from build123d import *

# Parameters (mm, degrees)
F1_ANGLE  = 180
F2_R      = 11
F3_DEPTH  = 3.5
F4_R      = 10.5
F5_DEPTH  = 17
F7_DEPTH  = 4
F8_R      = 18.641205443
F8_R_2    = 11
F9_DEPTH  = 4
F10_R     = 10
F11_DEPTH = 2
F13_DEPTH = 3
F15_DEPTH = 25
F17_DEPTH = 3
F18_R     = 2.5
F19_DEPTH = 2.5
F20_R     = 1.5
F21_DEPTH = 25


with BuildPart() as f1:
    # F0 (on Top) → F1 (revolve)
    with BuildSketch(Plane.XY):
        with BuildLine():
            ThreePointArc((0, -17.5), (12.3743686708, -12.3743686708), (17.5, 0))
            ThreePointArc((17.5, 0), (12.3743686708, 12.3743686708), (0, 17.5))
            Line((0, 17.5), (0, -17.5))
        make_face()
    revolve(axis=Axis((0, 0, 0), (0, -1, 0)), revolution_arc=F1_ANGLE)

    # F2 (on face) → F3 (cut)
    with BuildSketch(Plane(origin=(0, 0, 0), x_dir=(1, 0, 0), z_dir=(0, 0, -1))):
        Circle(F2_R)
    extrude(amount=-F3_DEPTH, mode=Mode.SUBTRACT)

    # F4 (on face) → F5 (cut)
    with BuildSketch(Plane(origin=(0, 0, 3.5), x_dir=(1, 0, 0), z_dir=(0, 0, -1))):
        Circle(F4_R)
    extrude(amount=-F5_DEPTH, mode=Mode.SUBTRACT)



with BuildPart() as f7:
    # F6 (on face) → F7 (new body)
    with BuildSketch(Plane(origin=(0, 0, 0), x_dir=(1, 0, 0), z_dir=(0, 0, -1))):
        with BuildLine():
            ThreePointArc((-12.3743686708, -12.3743686708), (-17.5, 0), (-12.3743686708, 12.3743686708))
            Line((-12.3743686708, 12.3743686708), (-14.1421356237, 14.1421356237))
            ThreePointArc((-14.1421356237, 14.1421356237), (-27.8923182516, 7.317919876), (-43.1821195756, 8.6815247843))
            Line((-43.1821195756, 8.6815247843), (-48.919726111, 4.6715533074))
            ThreePointArc((-48.919726111, 4.6715533074), (-34.6649635656, -10.5286316429), (-14.1421356237, -14.1421356237))
            Line((-14.1421356237, -14.1421356237), (-12.3743686708, -12.3743686708))
        make_face()
        with BuildLine():
            Line((-14.1421356237, 14.1421356237), (-12.3743686708, 12.3743686708))
            ThreePointArc((-12.3743686708, 12.3743686708), (0, 17.5), (12.3743686708, 12.3743686708))
            Line((12.3743686708, 12.3743686708), (14.1421356237, 14.1421356237))
            ThreePointArc((14.1421356237, 14.1421356237), (7.317919876, 27.8923182516), (8.6815247843, 43.1821195756))
            Line((8.6815247843, 43.1821195756), (4.6715533074, 48.919726111))
            ThreePointArc((4.6715533074, 48.919726111), (-10.5286316429, 34.6649635656), (-14.1421356237, 14.1421356237))
        make_face()
        with BuildLine():
            Line((14.1421356237, 14.1421356237), (12.3743686708, 12.3743686708))
            ThreePointArc((12.3743686708, 12.3743686708), (17.5, 0), (12.3743686708, -12.3743686708))
            Line((12.3743686708, -12.3743686708), (14.1421356237, -14.1421356237))
            ThreePointArc((14.1421356237, -14.1421356237), (27.8923182516, -7.317919876), (43.1821195756, -8.6815247843))
            Line((43.1821195756, -8.6815247843), (48.919726111, -4.6715533074))
            ThreePointArc((48.919726111, -4.6715533074), (34.6649635656, 10.5286316429), (14.1421356237, 14.1421356237))
        make_face()
        with BuildLine():
            ThreePointArc((12.3743686708, -12.3743686708), (0, -17.5), (-12.3743686708, -12.3743686708))
            Line((-12.3743686708, -12.3743686708), (-14.1421356237, -14.1421356237))
            ThreePointArc((-14.1421356237, -14.1421356237), (-7.317919876, -27.8923182516), (-8.6815247843, -43.1821195756))
            Line((-8.6815247843, -43.1821195756), (-4.6715533074, -48.919726111))
            ThreePointArc((-4.6715533074, -48.919726111), (10.5286316429, -34.6649635656), (14.1421356237, -14.1421356237))
            Line((14.1421356237, -14.1421356237), (12.3743686708, -12.3743686708))
        make_face()
    extrude(amount=-F7_DEPTH)


with BuildPart() as f1_1:
    add(f1.part)

    add(f7.part)  # F9 merges F7
    # F8 (on face) → F9 (join, through all)
    with BuildSketch(Plane(origin=(0, 0, 0), x_dir=(1, 0, 0), z_dir=(0, 0, -1))):
        Circle(F8_R)
        Circle(F8_R_2, mode=Mode.SUBTRACT)
    extrude(amount=-F9_DEPTH)

    # F10 (on face) → F11 (cut)
    with BuildSketch(Plane(origin=(0, 0, 0), x_dir=(1, 0, 0), z_dir=(0, 0, -1))):
        with Locations((-3.7499996834, 22.8846166283)):
            Circle(F10_R)
        with Locations((-22.8846166283, -3.7499996834)):
            Circle(F10_R)
        with Locations((3.7499996834, -22.8846166283)):
            Circle(F10_R)
        with Locations((22.8846166283, 3.7499996834)):
            Circle(F10_R)
    extrude(amount=-F11_DEPTH, mode=Mode.SUBTRACT)

    # F12 (on face) → F13 (cut)
    with BuildSketch(Plane(origin=(0, 0, 0), x_dir=(1, 0, 0), z_dir=(0, 0, -1))):
        Polygon((5.9440483259, 41.5129213729), (8.2390909401, 43.1169099636), (4.9165431449, 47.8709268072), (2.6215005308, 46.2669382165), (2.2936373002, 46.0377969892), (5.6161850953, 41.2837801456), align=None)
        Polygon((-46.0377969892, 2.2936373002), (-41.2837801456, 5.6161850953), (-41.5129213729, 5.9440483259), (-43.1169099636, 8.2390909401), (-47.8709268072, 4.9165431449), (-46.2669382165, 2.6215005308), align=None)
        Polygon((-2.2936373002, -46.0377969892), (-5.6161850953, -41.2837801456), (-5.9440483259, -41.5129213729), (-8.2390909401, -43.1169099636), (-4.9165431449, -47.8709268072), (-2.6215005308, -46.2669382165), align=None)
        Polygon((46.0377969892, -2.2936373002), (41.2837801456, -5.6161850953), (41.5129213729, -5.9440483259), (43.1169099636, -8.2390909401), (47.8709268072, -4.9165431449), (46.2669382165, -2.6215005308), align=None)
    extrude(amount=-F13_DEPTH, mode=Mode.SUBTRACT)

    # F14 (on face) → F15 (cut)
    with BuildSketch(Plane(origin=(0, 0, 0), x_dir=(1, 0, 0), z_dir=(0, 0, -1))):
        Polygon((5.7307557089, 41.1198485303), (2.2936373002, 46.0377969892), (2.20770934, 46.1607457007), (0.9782222253, 45.3014660985), (4.415340634, 40.3835176396), (4.5012685942, 40.2605689282), align=None)
        Polygon((-46.1607457007, 2.20770934), (-45.3014660985, 0.9782222253), (-40.3835176396, 4.415340634), (-40.2605689282, 4.5012685942), (-41.1198485303, 5.7307557089), (-46.0377969892, 2.2936373002), align=None)
        Polygon((-2.20770934, -46.1607457007), (-0.9782222253, -45.3014660985), (-4.415340634, -40.3835176396), (-4.5012685942, -40.2605689282), (-5.7307557089, -41.1198485303), (-2.2936373002, -46.0377969892), align=None)
        Polygon((46.1607457007, -2.20770934), (45.3014660985, -0.9782222253), (40.3835176396, -4.415340634), (40.2605689282, -4.5012685942), (41.1198485303, -5.7307557089), (46.0377969892, -2.2936373002), align=None)
    extrude(amount=-F15_DEPTH, mode=Mode.SUBTRACT)

    # F16 (on face) → F17 (cut)
    with BuildSketch(Plane(origin=(0, 0, 0), x_dir=(1, 0, 0), z_dir=(0, 0, -1))):
        with BuildLine():
            Line((4.1809628018, 40.7188735865), (1.342054472, 44.7808822767))
            ThreePointArc((1.342054472, 44.7808822767), (-5.3985401919, 39.5803016206), (-8.5350042844, 31.6654896468))
            ThreePointArc((-8.5350042844, 31.6654896468), (-4.3224338027, 32.8682191434), (0, 32.1548648652))
            ThreePointArc((0, 32.1548648652), (1.0537931887, 36.9429820748), (4.1809628018, 40.7188735865))
        make_face()
        with BuildLine():
            Line((-40.7188735865, 4.1809628018), (-44.7808822767, 1.342054472))
            ThreePointArc((-44.7808822767, 1.342054472), (-39.5803016206, -5.3985401919), (-31.6654896468, -8.5350042844))
            ThreePointArc((-31.6654896468, -8.5350042844), (-32.8682191434, -4.3224338027), (-32.1548648653, 0))
            ThreePointArc((-32.1548648653, 0), (-36.9429820748, 1.0537931887), (-40.7188735865, 4.1809628018))
        make_face()
        with BuildLine():
            Line((-4.1809628018, -40.7188735865), (-1.342054472, -44.7808822767))
            ThreePointArc((-1.342054472, -44.7808822767), (5.3985401919, -39.5803016206), (8.5350042844, -31.6654896468))
            ThreePointArc((8.5350042844, -31.6654896468), (4.3224338027, -32.8682191434), (0, -32.1548648653))
            ThreePointArc((0, -32.1548648653), (-1.0537931887, -36.9429820748), (-4.1809628018, -40.7188735865))
        make_face()
        with BuildLine():
            Line((40.7188735865, -4.1809628018), (44.7808822767, -1.342054472))
            ThreePointArc((44.7808822767, -1.342054472), (39.5803016206, 5.3985401919), (31.6654896468, 8.5350042844))
            ThreePointArc((31.6654896468, 8.5350042844), (32.8682191434, 4.3224338027), (32.1548648652, 0))
            ThreePointArc((32.1548648652, 0), (36.9429820748, -1.0537931887), (40.7188735865, -4.1809628018))
        make_face()
    extrude(amount=-F17_DEPTH, mode=Mode.SUBTRACT)

    # F18 (on face) → F19 (join)
    with BuildSketch(Plane(origin=(0, 0, 0), x_dir=(1, 0, 0), z_dir=(0, 0, -1))):
        with Locations((8.4528671578, 13.4043414146)):
            Circle(F18_R)
        with Locations((-13.4043414146, 8.4528671578)):
            Circle(F18_R)
        with Locations((-8.4528671578, -13.4043414146)):
            Circle(F18_R)
        with Locations((13.4043414146, -8.4528671578)):
            Circle(F18_R)
    extrude(amount=F19_DEPTH)

    # F20 (on face) → F21 (cut)
    with BuildSketch(Plane(origin=(0, 0, 0), x_dir=(1, 0, 0), z_dir=(0, 0, -1))):
        with Locations((4.0849614888, 34.4008803368)):
            Circle(F20_R)
        with Locations((-34.4008803368, 4.0849614888)):
            Circle(F20_R)
        with Locations((-4.0849614888, -34.4008803368)):
            Circle(F20_R)
        with Locations((34.4008803368, -4.0849614888)):
            Circle(F20_R)
    extrude(amount=-F21_DEPTH, mode=Mode.SUBTRACT)


solid = f1_1.part
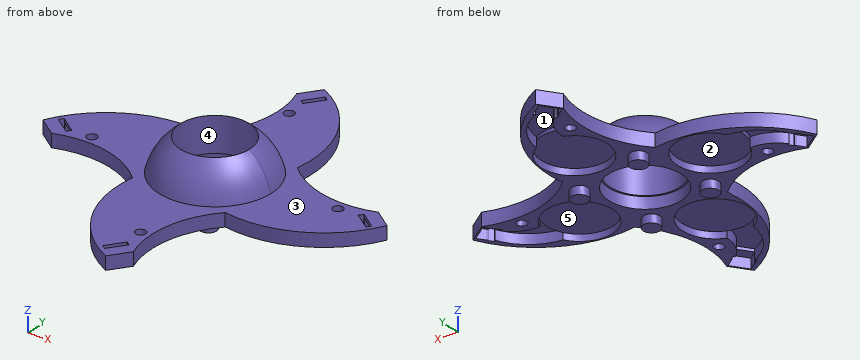
Here's how the part is built. I have some questions about the finished solid (model axes, mm). Face numbers are marked on the shaded views. A direction names the side the tool comes from. Coordinates: 2 decimals unless noted, no trailing zeros. Write each loop counter-clockwise with the first axis right and the second up, starting at its lowest first coordinate (ties: lowest second). Pieces come first, ordered by that corner, then holes.
1) Thinking about a two-plate mould opening in Y: for the marked faces 1, 2 and 3, which applies, +Y half, -Y half, draft (parallel to the pull), parting line (faces both ways), or undercut?
Filled in:
face 1: undercut
face 2: undercut
face 3: draft
2) I'm going to push flat-ended pins straight in: pin 1 (14 mm diameter, centred on x = -36, y = 4, fed in from -Z); pin 2 (8 mm diameter, centred on x = -33.5, z = 9, fed in from +Y); pin 3 (1.5 mm diameter, centred on x = -12.5, y = 11, fed in from +Z); pin 4 (5 mm diameter, centred on x = 4.08, y = -34.4, fed in from +Z). Where does each tip first touch, or does it pass through?
Filled in:
pin 1: stops at z = 0
pin 2: passes through
pin 3: stops at z = 7.31
pin 4: stops at z = 4
3) If we section it at B-B (y = 22): List the corners of the cut face in (x, z) for me.
Filled in:
outline: (-9.11, 0) - (-6.21, 0) - (-6.21, 2) - (13.71, 2) - (13.71, 0) - (14.36, 0) - (14.36, 4) - (-9.11, 4) - close
4) If I drill on line 1 (Y direction, x = 2.5, z = 1.75); line 2 (Z direction, x = 9.5, y = -21); line 3 (X direction, y = 3.75, z = 1.45), over which ranges is the centre line in solid material (lowest first)?
Filled in:
line 1: y = -47.82 to -46.18, -39.15 to -30.69, -15.08 to -10.71, 10.71 to 12.96, 42.54 to 44.42
line 2: z = 0 to 4
line 3: x = -43.33 to -41.45, -12.88 to -10.34, 10.34 to 16.27, 29.5 to 32.94, 35.86 to 40.38, 47.06 to 48.48
5) If we section it at D-D (z = 5.5): List the corners of the cut face in (x, y) for me, plus the area to 3 significant figures.
Filled in:
outline: circle Ø33.23 at (0, 0); hole circle Ø21 at (0, 0)
area: 521 mm2
6) If we section it at C-C (z = 11.5): List the corners of the cut face in (x, y) for me.
Filled in:
outline: circle Ø26.38 at (0, 0); hole circle Ø21 at (0, 0)
7) Which directions (+Z, -Z, +X, -X, +Y, -Y) give clear straight access to the entire face, cutting with the end or side of a thin tool? Please do the marked faces 4 and 5.
Filled in:
face 4: +Z, -Z
face 5: -Z
8) If we section it at A-A (x = -29.5): List the corners of the cut face in (y, z) for me, plus the area to 3 significant figures.
Filled in:
outline: (-7.06, 0) - (-3.75, 0) - (-3.75, 2) - (11.25, 2) - (11.25, 0) - (12.78, 0) - (12.78, 4) - (-7.06, 4) - close
area: 49.4 mm2
